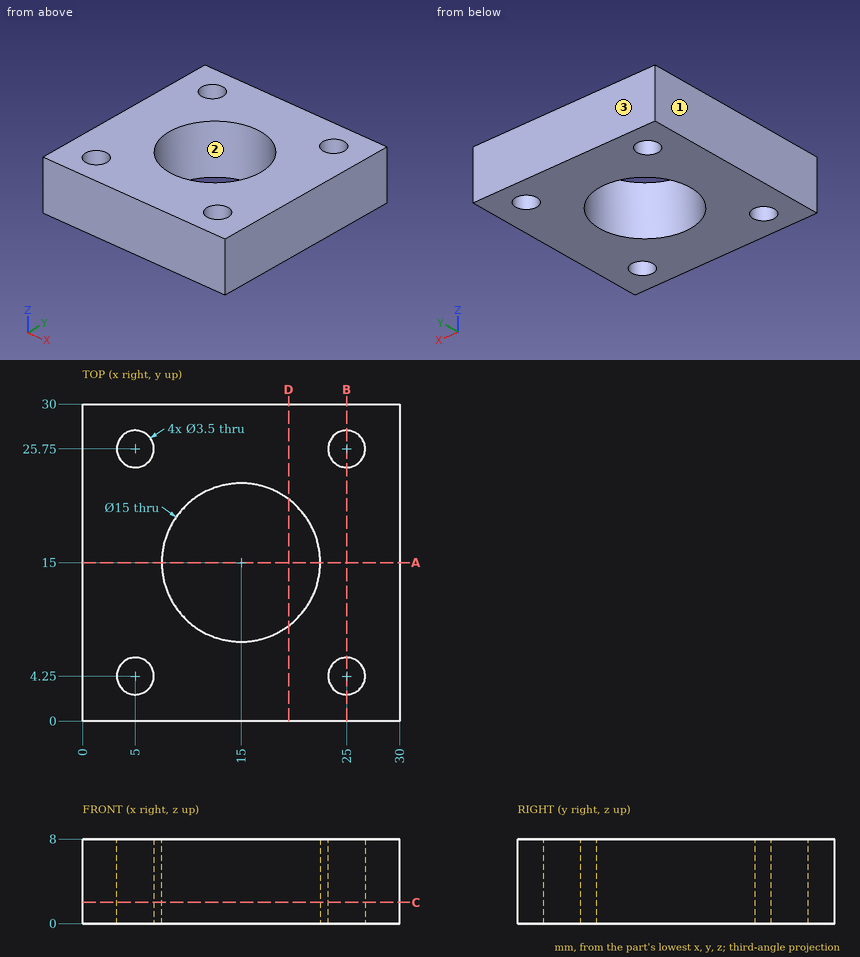
The figure shows three views and two pictorial views of one solid part (mm, origin at its lowest corner). Answer the questions. Round coordinates to 2 decimals unless told otherwise and drop trailing zeros. Loops run counter-clockwise (first coordinate to the right, second up) from the corner with the lowest first, then second, coordinate; pieces in that order, holes last. Notation, with made-up numbers: (40, -10.5) - (53, -10.5) arc R30 ccw to (53, 14.5) - close; hole circle Ø1 at (36.5, -28). An arc over 180 degrees is marked (long way). Use one line per item in the form item = value. Start each with the question number.
(1) Flat-ended cylindrical pins translate along their axes: P1, Ø3, axis at x = 25, y = 4.25, coming from the -Z side; P2, Ø6, axis at x = 5.5, y = 19.5, coming from the -Z side. Find the tip coordinate at first contact, or state that the pin passes through.
(2) Find section A-A on y = 15. Determine the outline of the cut face in (x, z), and give its area (3 significant figures).
(3) Find section B-B on x = 25. Determine the outline of the cut face in (y, z), and give its area (3 significant figures).
(4) Determine the mould class of the marked faces 1, 2 and 3 for opening direction Y: +Y half, -Y half, draft (parallel to the pull), parting line (faces both ways), or undercut.
(5) Find section D-D on x = 19.5. Determine the outline of the cut face in (y, z).
(6) Consider line 1 (Y direction, x = 5, z = 4); line 2 (Y direction, x = 24.25, z = 4); line 3 (Y direction, x = 12.25, z = 6.5). Determine where each line is inside the solid, lowest interval first.
(7) Find section C-C on z = 2. Determine the outline of the cut face in (x, y).
Answer list:
q1.P1 = through
q1.P2 = 0
q2.outline = (0, 0) - (7.5, 0) - (7.5, 8) - (0, 8) - close; (22.5, 0) - (30, 0) - (30, 8) - (22.5, 8) - close
q2.area = 120 mm^2
q3.outline = (0, 0) - (2.5, 0) - (2.5, 8) - (0, 8) - close; (6, 0) - (24, 0) - (24, 8) - (6, 8) - close; (27.5, 0) - (30, 0) - (30, 8) - (27.5, 8) - close
q3.area = 184 mm^2
q4.face_1 = draft
q4.face_2 = undercut
q4.face_3 = +Y half
q5.outline = (0, 0) - (9, 0) - (9, 8) - (0, 8) - close; (21, 0) - (30, 0) - (30, 8) - (21, 8) - close
q6.line_1 = 0 to 2.5, 6 to 24, 27.5 to 30
q6.line_2 = 0 to 2.67, 5.83 to 24.17, 27.33 to 30
q6.line_3 = 0 to 8.02, 21.98 to 30
q7.outline = (0, 0) - (30, 0) - (30, 30) - (0, 30) - close; hole circle Ø3.5 at (5, 4.25); hole circle Ø3.5 at (5, 25.75); hole circle Ø15 at (15, 15); hole circle Ø3.5 at (25, 4.25); hole circle Ø3.5 at (25, 25.75)
